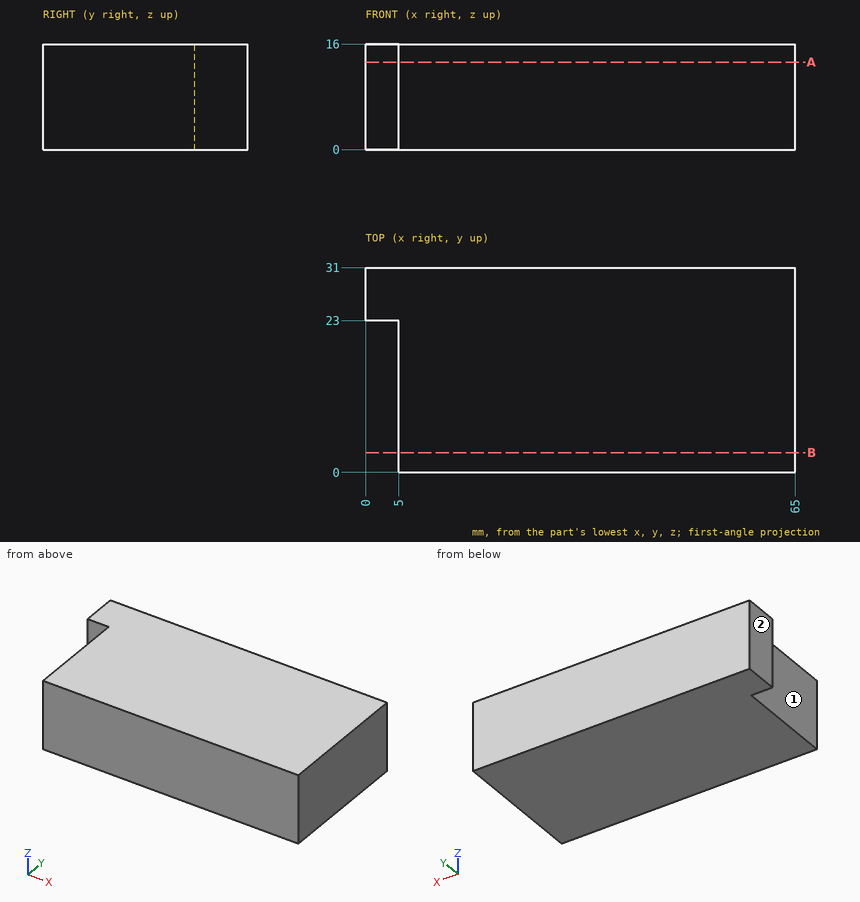
Input: dimensioned drawing with shaded views. Units: mm. Origin: part minimum x, y, z. A direction names the side the tool comes from. Give positions to 0.01 mm unless a question says otherwise; leave off trailing zeros. Write each loop counter-clockwise with the first axis right and the second up, starting at its lowest first coordinate (ties: lowest second). Pieces come first, ordered by that corner, then holes. Notation, with made-up numbers: (-34, 60.5) - (11, 60.5) arc R23 ccw to (11, 93.5) - close; hole circle Ø6 at (-27.5, 50.5). An arc over 180 degrees is marked (long way). One line per item, written item: value. Start each with the question number.
Q1. Set-up query: the marked faces 1 and 2. Return all of +Z, -Z, +X, -X, +Y, -Y with unobstructed straight access to the full face (end or side cutting, diameter ignored); none if empty.
Q2. Material intervals for probe 1 along X at (y, z) = (16.5, 6.5), sorted ascending. Write a range as from..to.
Q3. First-contact query: pin 1 Ø1.5 at (y, z) = (5.5, 8.5) entering from -X; pin 2 Ø4 at (x, z) = (1.5, 9.5) entering from -Y. Flat tips, straight axial feed; report the tip coordinate or a pass-through.
Q4. Section query B-B, the plane y = 3. Return the cut outline in (x, z), then the cut area to 3 significant figures.
Q5. Section query A-A, the plane z = 13.25. Return the cut outline in (x, y), then the cut area to 3 significant figures.
Answer:
1. face 1: +Z, -Z, -X, -Y
1. face 2: +Z, -Z, -X, +Y, -Y
2. probe 1: x = 5..65
3. pin 1: stops at x = 5
3. pin 2: stops at y = 23
4. outline: (5, 0) - (65, 0) - (65, 16) - (5, 16) - close
4. area: 960 mm2
5. outline: (0, 23) - (5, 23) - (5, 0) - (65, 0) - (65, 31) - (0, 31) - close
5. area: 1,900 mm2
